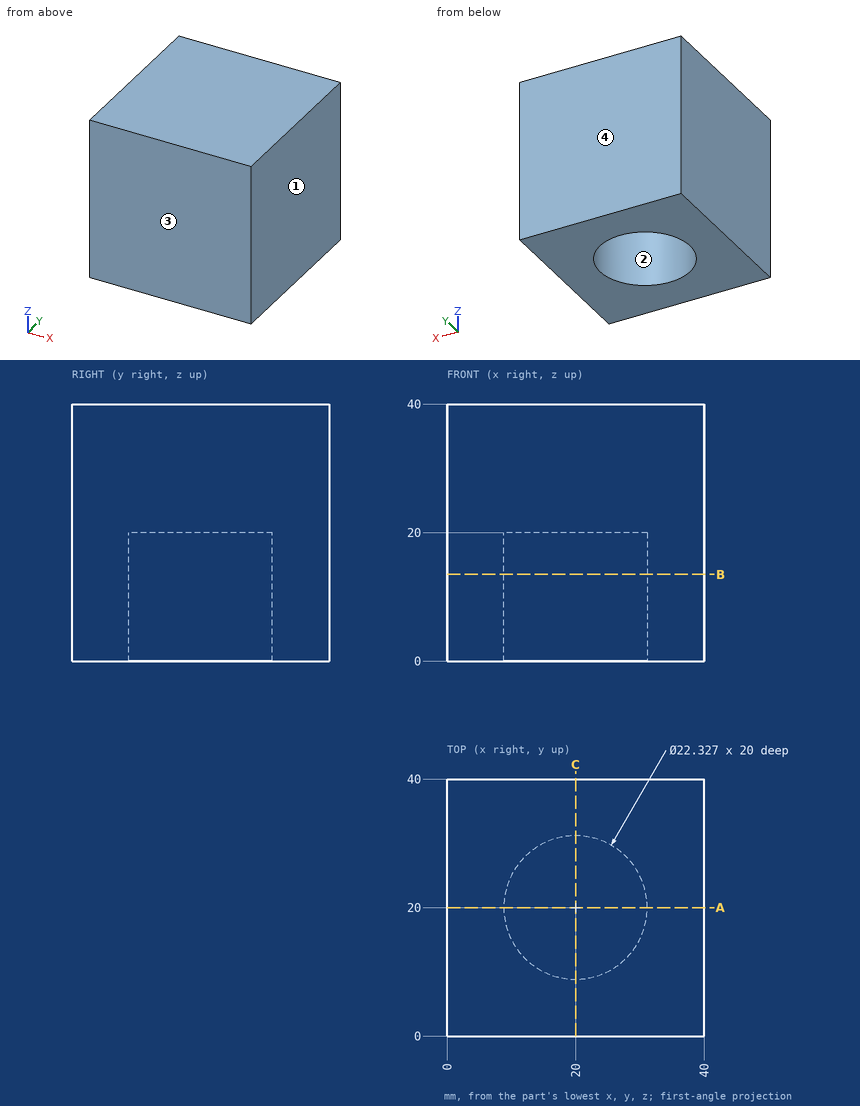
Geometry: see drawing. Coordinates: mm, zero at the bounding-box minimum. Give positions to 0.01 mm unless a question says otherwise; leave off trailing zeros. Loops run counter-clockwise (first coordinate to the right, second up) from the corner with the lowest first, then second, coordinate; pieces in that order, holes last. Notation, with made-up numbers: (84.5, 79) - (92.5, 79) arc R26 cw to (92.5, 93) - close; hole circle Ø3 at (15, -31). An arc over 180 degrees is marked (long way). One line per question, with ' | ' between items. Start each with the question number.
(1) Section query A-A on y = 20. Return loops of the section in (x, z), then the cut area to 3 significant figures.
(2) Section query B-B on z = 13.5. Return loops of the section in (x, y), then the cut area to 3 significant figures.
(3) Contact query for a flat-ended pin moving along its axis: pin 1 (11 mm diameter, centred on x = 21, y = 18, fed in from -Z). Output: stop coordinate, or through.
(4) Pull-direction query (Y, two-part tool) for the marked faces 1, 2, 3 and 4; classes: released by +Y, released by -Y, zero draft, split by the parting line, or undercut.
(5) Ray query, line 1 (Y direction, x = 20.5, z = 7); line 2 (Z direction, x = 21, y = 17.5); line 3 (X direction, y = 19, z = 8). Return the intervals inside material, ascending. Write a range as from..to.
The answers:
1) outline: (0, 0) - (8.84, 0) - (8.84, 20) - (31.16, 20) - (31.16, 0) - (40, 0) - (40, 40) - (0, 40) - close | area: 1,150 mm2
2) outline: (0, 0) - (40, 0) - (40, 40) - (0, 40) - close; hole circle Ø22.33 at (20, 20) | area: 1,210 mm2
3) pin 1: z = 20
4) face 1: zero draft | face 2: undercut | face 3: released by -Y | face 4: released by +Y
5) line 1: 0..8.85, 31.15..40 | line 2: 20..40 | line 3: 0..8.88, 31.12..40
